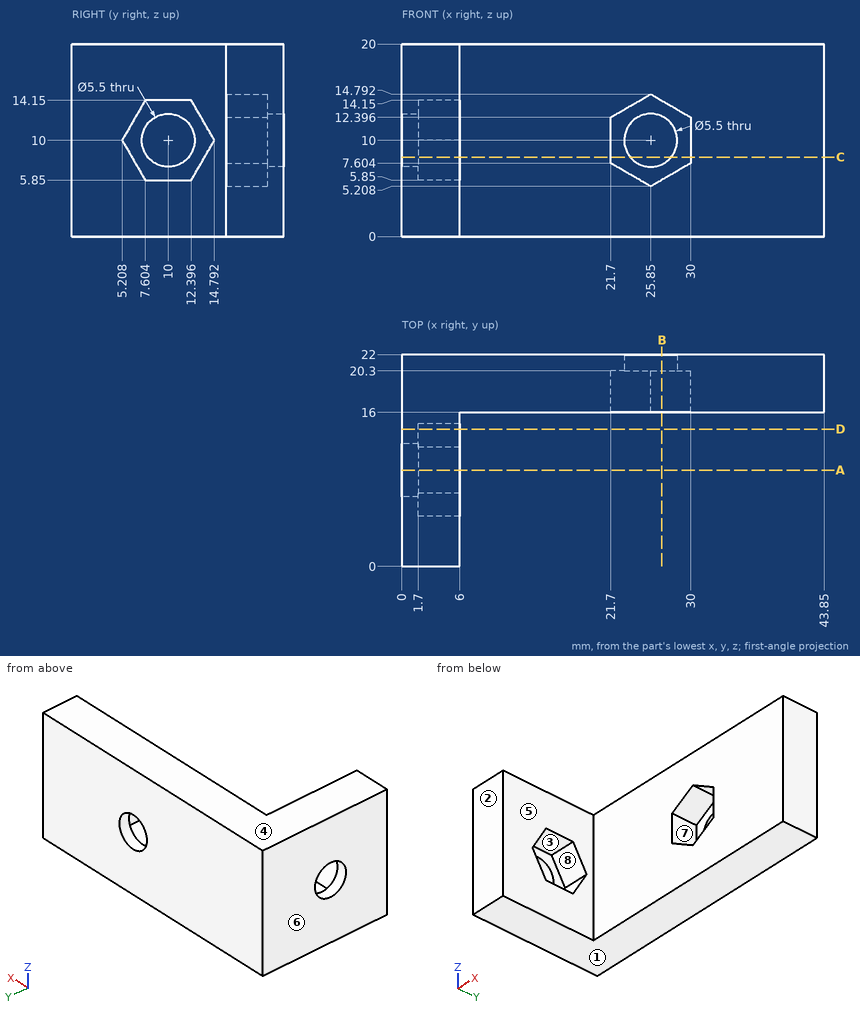
Drawing for the job (mm, zero at the part's lowest x, y, z). A direction names the side the tool comes from. Round coordinates to 2 decimals unless told otherwise and drop trailing zeros. Loops run counter-clockwise (first coordinate to the right, second up) from the corner with the lowest first, then second, coordinate; pieces in that order, holes last.
1. Wall check: probe 1 along X at (y, z) = (20.7, 10); probe 2 along Y at (x, z) = (0.85, 10); probe 3 along X at (y, z) = (16.75, 10.25). Give the ranges that are in metal, low to high.
Check values:
probe 1: x = 0 to 23.1, 28.6 to 43.85
probe 2: y = 0 to 7.25, 12.75 to 22
probe 3: x = 0 to 21.7, 30 to 43.85
2. Drop flat-ended pins along their axis: P1, Ø1.5, axis at x = 6.5, y = 7, coming from the -Z side; P2, Ø1, axis at y = 12, z = 15, coming from the +X side; P3, Ø9, axis at x = 24, z = 8, coming from the -Y side; P4, Ø5, axis at x = 25.85, z = 10, coming from the +Y side. Give the stop position or say it passes through.
Check values:
P1: stops at z = 0
P2: stops at x = 6
P3: stops at y = 16
P4: passes through
3. Mould opens along Y. For the marked faces 1, 2 and 3 say: +Y half, -Y half, draft (parallel to the pull), parting line (faces both ways), or undercut.
Check values:
face 1: draft
face 2: -Y half
face 3: undercut
4. Tool access for the marked faces 4, 5, 6, 7 and 8: list every direction of +Z, -Z, +X, -X, +Y, -Y with a clear straight run to the whole face (end or side of a thin tool).
Check values:
face 4: +Z, +X, -X, +Y, -Y
face 5: +Z, -Z, +X, -Y
face 6: +Z, -Z, -X, +Y, -Y
face 7: -Y
face 8: +X
5. Band-saw the part on D-D, the plane y = 14.25. List the corners of the cut face in (x, z).
Check values:
outline: (0, 0) - (6, 0) - (6, 9.06) - (1.7, 9.06) - (1.7, 10.94) - (6, 10.94) - (6, 20) - (0, 20) - close
6. Band-saw the part on B-B, the plane x = 27. List the corners of the cut face in (y, z), and give its area (3 significant figures).
Check values:
outline: (16, 0) - (22, 0) - (22, 7.5) - (20.3, 7.5) - (20.3, 5.87) - (16, 5.87) - close; (16, 14.13) - (20.3, 14.13) - (20.3, 12.5) - (22, 12.5) - (22, 20) - (16, 20) - close
area: 76.0 mm2
7. Band-saw the part on C-C, the plane z = 8.25. List the corners of the cut face in (x, y).
Check values:
outline: (0, 0) - (6, 0) - (6, 6.22) - (1.7, 6.22) - (1.7, 7.88) - (0, 7.88) - close; (0, 12.12) - (1.7, 12.12) - (1.7, 13.78) - (6, 13.78) - (6, 16) - (21.7, 16) - (21.7, 20.3) - (23.73, 20.3) - (23.73, 22) - (0, 22) - close; (27.97, 20.3) - (30, 20.3) - (30, 16) - (43.85, 16) - (43.85, 22) - (27.97, 22) - close
8. Band-saw the part on A-A, the plane y = 10. List the corners of the cut face in (x, z), and give its area (3 significant figures).
Check values:
outline: (0, 0) - (6, 0) - (6, 5.85) - (1.7, 5.85) - (1.7, 7.25) - (0, 7.25) - close; (0, 12.75) - (1.7, 12.75) - (1.7, 14.15) - (6, 14.15) - (6, 20) - (0, 20) - close
area: 75.0 mm2
